Geometry check sheet. Reference: the model listing, model coordinates, mm. Face numbers are marked on the shaded views. Round coordinates to 2 decimals unless told otherwise and drop trailing zeros. Order: outer loops, then holes, each group sorted by start corner. A loop starts at its lowest first (then second) coordinate and runs counter-clockwise, first axis right, second up. Notation, with made-up numbers: (21.25, 75.5) - (26.25, 75.5) arc R18 cw to (26.25, 80.5) - close; hole circle Ø3 at (-24.5, 82.25). An arc over 180 degrees is marked (long way). Return JSON: item names as keys, results as strings. Group by question number.
Q1. Sectioned sample at B-B, the plane z = 44.45. Record the cut outline in (x, y) (3 decimals), then the cut area to 3 significant figures.
Q2. Sectioned sample at D-D, the plane x = 28. Record the cut outline in (y, z).
Q3. Sectioned sample at C-C, the plane z = 28. Record the cut outline in (x, y) (3 decimals).
Q4. Material ranges on line 1 along Y through (x, z) = (0, 36) (3 decimals); line 2 along Y through (x, z) = (44, 43); line 3 along Y through (x, z) = (4, 26.5), recorded low to high.
Q5. Sectioned sample at A-A, the plane x = 0. Record the cut outline in (y, z) (3 decimals), then the cut area to 3 significant figures.
Q6. Gauge pin test, flat ends, axial feed: pin 1 Ø6 at (y, z) = (6.5, 9) entering from +X; pin 2 Ø21 at (x, z) = (31.71, 19.05) entering from +Y; pin 3 Ø5 at (x, z) = (10.5, 56) entering from -Y. Record the tip position at first contact, or that the pin passes through.
Q7. Draft check along Y on the marked faces 1, 2 and 3. Enter one of: pulls with the +Y half, pulls with the -Y half, needs draft (parallel to the pull), parting line crosses it, or undercut.
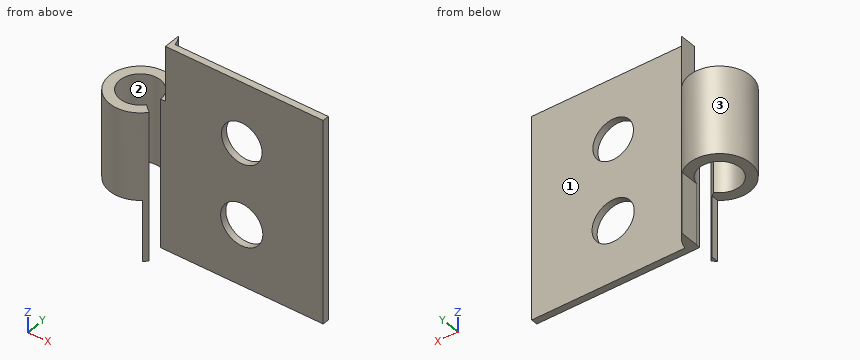
```python
from build123d import *

# Parameters (mm, degrees)
F1_DEPTH = 63.5
F2_R     = 6.35
F2_R_2   = 6.589045
F3_DEPTH = 9.526
F4_W     = 29.302539
F4_H     = 19.05
F4_W_2   = 28.424359
F5_DEPTH = 12.7


with BuildPart() as f1:
    # F0 (on Top) → F1 (new body)
    with BuildSketch(Plane.XY):
        with BuildLine():
            ThreePointArc((4.965456, -3.958124), (-5.993878, 2.096646), (6.35, 0))
            Line((6.35, 0), (57.15, 0))
            Line((57.15, 0), (57.15, 2.05693))
            Line((57.15, 2.05693), (9.300251, 2.05693))
            ThreePointArc((9.300251, 2.05693), (-9.272442, 2.178863), (7.410832, -5.983744))
            Line((7.410832, -5.983744), (4.965456, -3.958124))
        make_face()
    extrude(amount=F1_DEPTH)

    # F2 (on face) → F3 (cut, through all)
    with BuildSketch(Plane.XZ):
        with Locations((31.714201, 44.45)):
            Circle(F2_R)
        with Locations((31.714201, 19.05)):
            Circle(F2_R_2)
    extrude(amount=-F3_DEPTH, mode=Mode.SUBTRACT)

    # F4 (on face) → F5 (cut, symmetric)
    with BuildSketch(Plane.XZ):
        with Locations((-8.445638, 9.525)):
            Rectangle(F4_W, F4_H)
        with Locations((-6.318135, 55.88594)):
            Rectangle(F4_W_2, F4_H)
    extrude(amount=F5_DEPTH, both=True, mode=Mode.SUBTRACT)


solid = f1.part
```
Reply:
{
 "1": {"outline": "(4.965, -3.958) arc R6.35 cw (long way) to (6.35, 0) - (25.364, 0) - (25.364, 2.057) - (9.3, 2.057) arc R9.525 ccw (long way) to (7.411, -5.984) - close; (38.064, 0) - (57.15, 0) - (57.15, 2.057) - (38.064, 2.057) - close", "area": "213 mm^2"},
 "2": {"outline": "(0, 0) - (2.06, 0) - (2.06, 13.61) - (0, 13.61) - close; (0, 24.49) - (2.06, 24.49) - (2.06, 39.3) - (0, 39.3) - close; (0, 49.6) - (2.06, 49.6) - (2.06, 63.5) - (0, 63.5) - close"},
 "3": {"outline": "(4.965, -3.958) arc R6.35 cw (long way) to (6.35, 0) - (57.15, 0) - (57.15, 2.057) - (9.3, 2.057) arc R9.525 ccw (long way) to (7.411, -5.984) - close"},
 "4": {"line 1": "-9.525 to -6.35, 6.35 to 9.525", "line 2": "0 to 2.06", "line 3": "-8.64 to -4.93, 4.93 to 8.64"},
 "5": {"outline": "(-9.525, 19.05) - (-6.35, 19.05) - (-6.35, 46.361) - (-9.525, 46.361) - close; (6.35, 19.05) - (9.525, 19.05) - (9.525, 46.361) - (6.35, 46.361) - close", "area": "173 mm^2"},
 "6": {"pin 1": "x = 8.86", "pin 2": "y = 2.06", "pin 3": "y = 0"},
 "7": {"face 1": "pulls with the +Y half", "face 2": "undercut", "face 3": "parting line crosses it"}
}
